For this review, take the finished solid that the model builds, in its own axes (mm). A direction names the side the tool comes from. Round coordinates to 2 decimals unless told otherwise and drop trailing zeros. Order: outer loops, then holes, each group sorted by start corner. A loop starts at its lowest first (then second) coordinate and runs counter-clockwise, first axis right, second up. Notation, with made-up numbers: (-12, 53) -> (6, 53) arc R33 cw to (6, 90) -> close; hole circle Ø11 at (51.5, 1.5). An arc over 180 degrees is marked (long way). Use a Markdown table: item, result. Add a question column.
1) Consider section B-B (y = 25.5). State the section outline as (x, z) points, plus the area to 3 significant figures.
2) Wall thickness on line 1 along Z through (x, y) = (-81, 17.5); line 2 along Z through (x, y) = (14.5, 32); line 3 along X through (y, z) = (26, 7.5): over which ranges is each line inside the solid? List them lowest first. Write a range as [from, to].
3) Machinability: for faces 4 (the face through (25, 24, 6.4)), 5 (the face through (-115, 24, 6.5)), 6 (the face through (25, 12.6, 4)), which of the approach directions +Z, -Z, +X, -X, +Y, -Y give a long, thin tool a straight path to every point of the face, cutting with its end or side? Answer none if there is none.
4) Clearance check with flat-ended pins moving along their axes: P1, Ø2.5, axis at x = 14, z = 3.5, coming from the +Y side; P2, Ø1.5, axis at x = -95, y = 9.5, coming from the -Z side; P3, Ø1.4, axis at x = 27.5, z = 5, coming from the -Y side; P4, Ø4, axis at x = -111.5, z = 3.5, coming from the -Y side. State where each tip first meets the part, or that it passes through.
5) Consider section D-D (y = 37.5). State the section outline as (x, z) points, plus the area to 3 significant figures.
6) Draft analysis for pull direction Y (two halves, no side actions). For faces 1 (the face through (25, 24, 1.6)), 2 (the face through (-80, 24, 4)), 3 (the face through (-76.05, 7.605, 1.972)), state which applies: pulls with the +Y half, pulls with the -Y half, needs draft (parallel to the pull), parting line crosses it, or undercut.
```python
from build123d import *

# Parameters (mm, degrees)
F0_W     = 150
F0_H     = 40
F1_DEPTH = 8
F2_SIZE2 = 14.99999
F2_SIZE  = 3.99999
F4_DEPTH = 70
F6_DEPTH = 50


# Not quite as in the source:
# - a fillet or chamfer is up to 0.001 mm smaller than in the source, because OpenCascade refuses the exact size


with BuildPart() as f1:
    # F0 (on Top) → F1 (new body)
    with BuildSketch(Plane.XY):
        with Locations((-75, 20)):
            Rectangle(F0_W, F0_H)
    extrude(amount=F1_DEPTH)

    # F2 (size 4 and 15 in the source; OpenCascade refuses exactly that, so slightly less here)
    f2_edges = [f1.edges().sort_by_distance(p)[0] for p in [
        (-75, 0, 8),
        (-75, 0, 0),
    ]]
    f2_side = f1.faces().sort_by_distance((-75, 0, 4))[0]
    chamfer(f2_edges, length=F2_SIZE, length2=F2_SIZE2, reference=f2_side)

    # F3 (on face) → F4 (cut)
    with BuildSketch(Plane(origin=(-150, 0, 0), x_dir=(0, -1, 0), z_dir=(-1, 0, 0))):
        Polygon((-12.5, 1.5), (-12.5, 4), (-12.5, 6.5), (-35, 6.5), (-35, 1.5), align=None)
    extrude(amount=-F4_DEPTH, mode=Mode.SUBTRACT)

    # F5 (on face) → F6 (join)
    with BuildSketch(Plane.YZ):
        Polygon((12.6, 6.4), (12.6, 4), (12.6, 1.6), (34.9, 1.6), (34.9, 6.4), align=None)
    extrude(amount=F6_DEPTH)


solid = f1.part
```
Results list:
| question | item | result |
|---|---|---|
| 1 | outline | (-150, 0) -> (0, 0) -> (0, 1.6) -> (50, 1.6) -> (50, 6.4) -> (0, 6.4) -> (0, 8) -> (-150, 8) -> (-150, 6.5) -> (-80, 6.5) -> (-80, 1.5) -> (-150, 1.5) -> close |
| 1 | area | 1,090 mm2 |
| 2 | line 1 | [0, 1.5], [6.5, 8] |
| 2 | line 2 | [1.6, 6.4] |
| 2 | line 3 | [-150, 0] |
| 3 | face 4 | +Z, +X, +Y, -Y |
| 3 | face 5 | -X |
| 3 | face 6 | +Z, -Z, +X, -Y |
| 4 | P1 | y = 34.9 |
| 4 | P2 | z = 1.27 |
| 4 | P3 | y = 12.6 |
| 4 | P4 | y = 0 |
| 5 | outline | (-150, 0) -> (0, 0) -> (0, 8) -> (-150, 8) -> close |
| 5 | area | 1,200 mm2 |
| 6 | face 1 | needs draft |
| 6 | face 2 | undercut |
| 6 | face 3 | pulls with the -Y half |
